Solid Edge part; units mm, degrees
sketch "Sketch1" plane through (0, 0, 0) normal (0, 0, 1) x (1, 0, 0)
  circle A0 centre (0, 0) radius 3
extrude "Protrusion1" add sketch "Sketch1" along normal blind 1.7
sketch "Sketch2" plane through (0, 0, 0) normal (0, 0, -1) x (1, 0, 0)
  circle A0 centre (0, 0) radius 1.5
extrude "Protrusion2" add sketch "Sketch2" along normal blind 14.3
sketch "Sketch3" plane through (0, 0, -14.3) normal (0, 0, -1) x (1, 0, 0)
  circle A0 centre (0, 0) radius 1.4997
extrude "Cutout1" cut sketch "Sketch3" against normal blind 12 flip side to cut
chamfer "Chamfer_1" distance 0.225 angle 45 1 edges at (-1.4997, 0, -14.3)
sketch "Sketch4" plane through (0, 0, 1.7) normal (0, 0, 1) x (1, 0, 0)
  line L0 (-0.5774, 1) -> (0.5774, 1)
  line L1 (1.1547, 0) -> (0.5774, 1)
  line L2 (0.5774, -1) -> (1.1547, 0)
  line L3 (-0.5774, -1) -> (0.5774, -1)
  line L4 (-1.1547, 0) -> (-0.5774, -1)
  line L5 (-0.5774, 1) -> (-1.1547, 0)
extrude "Cutout2" cut sketch "Sketch4" against normal blind 1.1333
sketch "Sketch5" plane through (0, 0, 0) normal (0, -1, 0) x (1, 0, 0)
  line L0 (3, 1.7) -> (1.3, 0)
  line L1 (1.3, 0) -> (3, 0)
  line L2 (3, 0) -> (3, 1.7)
revolve "RevolvedCutout1" cut sketch "Sketch5" angle 360 about axis through (0, 0, 14.0017) along (0, 0, -1)
properties part number "24104634"
Work out the finished part from the listing and answer in its coordinate system (mm). A direction names the side the tool comes from. Give positions to 0.01 mm unless a question says otherwise; leave off trailing zeros. Loops run counter-clockwise (first coordinate to the right, second up) from the corner with the lowest first, then second, coordinate; pieces in that order, holes last. Notation, with made-up numbers: (-22, 60.5) -> (28, 60.5) arc R24 cw to (28, 87.5) -> close; hole circle Ø11 at (20, 77.5). An arc over 180 degrees is marked (long way). Use a Markdown table: item, result. Add a question column.
1. Flat-ended cylindrical pins translate along their axes: pin 1 Ø1.2 at (x, z) = (0, 1.5) entering from +Y; pin 2 Ø1.5 at (x, y) = (-1.5, 2) entering from -Z. Find the tip coordinate at first contact, or state that the pin passes through.
2. Find the intervals of material crossed by probe 1 along Z at (x, y) = (0.25, -0.65); probe 2 along Y at (x, z) = (0.1, -9); probe 3 along Y at (x, z) = (0.7, -6.25), in increasing order.
3. Section B-B on z = -1 is taken. Determine the outline of the cut face in (x, y), and give its area (3 significant figures).
4. Determine the mould class of faces 4 (the flat face through (0.87, 0.49, 1.14)), 5 (the cylindrical face through (-0.325, 1.464, -8.27)), 6 (the flat face through (-0.87, -0.49, 1.14)), 7 (the flat face through (0, -1.3, 1.7)) for opening direction Y: released by +Y, released by -Y, zero draft, split by the parting line, or undercut.
5. For faces 1 (the cylindrical face through (-1.5, 0.07, -1.13)), 2 (the flat face through (0, 1, 1)), 3 (the flat face through (0, 0, -14.3)), determine the directions among +Z, -Z, +X, -X, +Y, -Y from which every point of the face is accessible in a straight line to the end or side of a thin tool.
Results below:
| question | item | result |
|---|---|---|
| 1 | pin 1 | stops at y = 3 |
| 1 | pin 2 | stops at z = 0.45 |
| 2 | probe 1 | z = -14.3 to 0.57 |
| 2 | probe 2 | y = -1.5 to 1.5 |
| 2 | probe 3 | y = -1.33 to 1.33 |
| 3 | outline | circle Ø3 at (0, 0) |
| 3 | area | 7.07 mm^2 |
| 4 | face 4 | undercut |
| 4 | face 5 | split by the parting line |
| 4 | face 6 | undercut |
| 4 | face 7 | zero draft |
| 5 | face 1 | -Z |
| 5 | face 2 | +Z |
| 5 | face 3 | -Z, +X, -X, +Y, -Y |
